Read the model definition and answer for the solid it produces. Units are mm, in the model's axes. A direction names the side the tool comes from. Give positions to 0.01 mm unless a question says otherwise; leave off trailing zeros. Write each loop counter-clockwise with the first axis right and the second up, starting at its lowest first coordinate (ties: lowest second). Pieces come first, ordered by that corner, then holes.
```python
from build123d import *

# Parameters (mm, degrees)
SKETCH_1_W          = 96
SKETCH_1_H          = 70
EXTRUDE_1_DEPTH     = 10
FILLET_1_R          = 10
SKETCH_2_R          = 2.12
CUT_EXTRUDE_1_DEPTH = 10
SKETCH_3_R          = 5
CUT_EXTRUDE_2_DEPTH = 5
SKETCH_4_R          = 3.1
CUT_EXTRUDE_3_DEPTH = 5
CHAMFER_1_SIZE      = 1
CHAMFER_2_SIZE      = 2
SKETCH_5_W          = 50
SKETCH_5_H          = 30
CUT_EXTRUDE_4_DEPTH = 10
FILLET_2_R          = 10
CHAMFER_3_SIZE      = 2


with BuildPart() as part:
    # 草图1 → 凸台-拉伸1 (new body)
    with BuildSketch(Plane.XY):
        Rectangle(SKETCH_1_W, SKETCH_1_H)
    extrude(amount=EXTRUDE_1_DEPTH)

    # 圆角1
    fillet_1_edges = [part.edges().sort_by_distance(p)[0] for p in [
        (48, -35, 5),
        (-48, -35, 5),
        (-48, 35, 5),
        (48, 35, 5),
    ]]
    fillet(fillet_1_edges, radius=FILLET_1_R)

    # 草图2 → 切除-拉伸1 (cut)
    with BuildSketch(Plane.XY.offset(10)):
        with Locations((0, 25.5)):
            Circle(SKETCH_2_R)
        with Locations((-12.7, 25.5)):
            Circle(SKETCH_2_R)
        with Locations(Location((12.7, 25.5, 0), (0, 0, 180))):
            Circle(SKETCH_2_R)
        with Locations((-12.7, -25.5)):
            Circle(SKETCH_2_R)
        with Locations((0, -25.5)):
            Circle(SKETCH_2_R)
        with Locations((12.7, -25.5)):
            Circle(SKETCH_2_R)
    extrude(amount=-CUT_EXTRUDE_1_DEPTH, mode=Mode.SUBTRACT)

    # 草图3 → 切除-拉伸2 (cut)
    with BuildSketch(Plane.XY.offset(10)):
        with Locations((-38, 25)):
            Circle(SKETCH_3_R)
        with Locations((-38, 0)):
            Circle(SKETCH_3_R)
        with Locations((-38, -25)):
            Circle(SKETCH_3_R)
        with Locations(Location((38, -25, 0), (0, 0, 180))):
            Circle(SKETCH_3_R)
        with Locations(Location((38, 0, 0), (0, 0, 180))):
            Circle(SKETCH_3_R)
        with Locations(Location((38, 25, 0), (0, 0, 180))):
            Circle(SKETCH_3_R)
    extrude(amount=-CUT_EXTRUDE_2_DEPTH, mode=Mode.SUBTRACT)

    # 草图4 → 切除-拉伸3 (cut)
    with BuildSketch(Plane.XY.offset(5)):
        with Locations((-38, 25)):
            Circle(SKETCH_4_R)
        with Locations((-38, 0)):
            Circle(SKETCH_4_R)
        with Locations((-38, -25)):
            Circle(SKETCH_4_R)
        with Locations((38, 25)):
            Circle(SKETCH_4_R)
        with Locations((38, 0)):
            Circle(SKETCH_4_R)
        with Locations((38, -25)):
            Circle(SKETCH_4_R)
    extrude(amount=-CUT_EXTRUDE_3_DEPTH, mode=Mode.SUBTRACT)

    # 倒角1
    chamfer_1_edges = [part.edges().sort_by_distance(p)[0] for p in [
        (34.9, 0, 0),
        (34.9, -25, 0),
        (-41.1, 25, 0),
        (-41.1, 0, 0),
        (-41.1, -25, 0),
        (34.9, 25, 0),
    ]]
    chamfer(chamfer_1_edges, length=CHAMFER_1_SIZE)

    # 倒角2
    chamfer_2_edges = [part.edges().sort_by_distance(p)[0] for p in [
        (0, 35, 10),
        (48, 0, 10),
        (-48, 0, 10),
        (0, -35, 10),
        (-45.071067812, -32.071067812, 10),
        (45.071067812, -32.071067812, 10),
        (-45.071067812, 32.071067812, 10),
        (45.071067812, 32.071067812, 10),
    ]]
    chamfer(chamfer_2_edges, length=CHAMFER_2_SIZE)

    # 草图5 → 切除-拉伸4 (cut)
    with BuildSketch(Plane.XY.offset(10)):
        Rectangle(SKETCH_5_W, SKETCH_5_H)
    extrude(amount=-CUT_EXTRUDE_4_DEPTH, mode=Mode.SUBTRACT)

    # 圆角2
    fillet_2_edges = [part.edges().sort_by_distance(p)[0] for p in [
        (25, 15, 5),
        (25, -15, 5),
        (-25, -15, 5),
        (-25, 15, 5),
    ]]
    fillet(fillet_2_edges, radius=FILLET_2_R)

    # 倒角3
    chamfer_3_edges = [part.edges().sort_by_distance(p)[0] for p in [
        (25, 0, 10),
        (25, 0, 0),
        (0, -15, 10),
        (0, -15, 0),
        (0, 15, 10),
        (0, 15, 0),
        (-25, 0, 10),
        (-25, 0, 0),
        (22.071067812, -12.071067812, 10),
        (22.071067812, -12.071067812, 0),
        (22.071067812, 12.071067812, 10),
        (22.071067812, 12.071067812, 0),
        (-22.071067812, -12.071067812, 10),
        (-22.071067812, -12.071067812, 0),
        (-22.071067812, 12.071067812, 10),
        (-22.071067812, 12.071067812, 0),
    ]]
    chamfer(chamfer_3_edges, length=CHAMFER_3_SIZE)


solid = part.part
```
Item 1: Which of the six approach directions +Z, -Z, +X, -X, +Y, -Y give full straight-line access (tool end or side, diameter ignored) to faces 4 (the conical face through (22.39, -12.56, 8.57)), 5 (the cylindrical face through (-14.82, 25.59, 5.07)), 6 (the conical face through (-22.372, 12.536, 1.458))?
Result set:
face 4: +Z
face 5: +Z, -Z
face 6: -Z
Item 2: Section B-B (x = -12.7) is taken. Write down the section's boundary in (y, z).
Result set:
outline: (-35, 0) - (-27.62, 0) - (-27.62, 10) - (-33, 10) - (-35, 8) - close; (-23.38, 0) - (-17, 0) - (-15, 2) - (-15, 8) - (-17, 10) - (-23.38, 10) - close; (15, 2) - (17, 0) - (23.38, 0) - (23.38, 10) - (17, 10) - (15, 8) - close; (27.62, 0) - (35, 0) - (35, 8) - (33, 10) - (27.62, 10) - close
Item 3: Determine the mould class of faces 1 (the cylindrical face through (-21.99, -12.15, 4.96)), 2 (the cylindrical face through (44.99, -32.15, 4.06)), 3 (the flat face through (-48, 0, 4)) for opening direction Y: pulls with the +Y half, pulls with the -Y half, needs draft (parallel to the pull), parting line crosses it, or undercut.
Result set:
face 1: undercut
face 2: pulls with the -Y half
face 3: needs draft
Item 4: Each of these flat-tipped pins is pushed along its axis until it touches: pin 1 Ø3 at (x, y) = (37, 24) entering from +Z; pin 2 Ø9 at (x, y) = (38, -25) entering from +Z. Where does it stop, or does it pass through?
Result set:
pin 1: passes through
pin 2: stops at z = 5
Item 5: Find the intervals of material crossed by line 1 along Y through (x, z) = (-38, 7.1); line 2 along Y through (x, z) = (0, 3.75); line 3 along X through (y, z) = (-27, 0.5), in increasing order.
Result set:
line 1: y = -35 to -30, -20 to -5, 5 to 20, 30 to 35
line 2: y = -35 to -27.62, -23.38 to -15, 15 to 23.38, 27.62 to 35
line 3: x = -47.8 to -40.99, -35.01 to -14.2, -11.2 to -1.5, 1.5 to 11.2, 14.2 to 35.01, 40.99 to 47.8
Item 6: Section A-A (y = 0) is taken. Give the number of separate pieces and of enclosed holes in the cut face, and give its area (3 significant figures).
Result set:
separate pieces: 4
enclosed holes: 0
area: 284 mm2
